from build123d import *

# Parameters (mm, degrees)
SKETCH1_R                                 = 74.5363
SKETCH1_R_2                               = 73.2663
BOSS_EXTRUDE1_DEPTH                       = 19.05
F_1_4_0_25_DIAMETER_HOLE1_REACH           = 179.139
F_1_4_0_25_DIAMETER_HOLE1_BORE_R          = 3.175
F_1_4_0_25_DIAMETER_HOLE1_ON_FACE_2_REACH = 179.139
F_1_4_0_25_DIAMETER_HOLE1_BORE_2_R        = 3.175
F_1_4_0_25_DIAMETER_HOLE4_REACH           = 168.94
F_1_4_0_25_DIAMETER_HOLE4_BORE_R          = 3.175
F_1_4_0_25_DIAMETER_HOLE4_ON_FACE_2_REACH = 168.949
F_1_4_0_25_DIAMETER_HOLE4_BORE_2_R        = 3.175
F_1_4_0_25_DIAMETER_HOLE4_ON_FACE_3_REACH = 168.94
F_1_4_0_25_DIAMETER_HOLE4_BORE_3_R        = 3.175


with BuildPart() as part:
    # Sketch1 → Boss-Extrude1 (new body)
    with BuildSketch(Plane(origin=(0, 0, 0), x_dir=(1, 0, 0), z_dir=(0, 1, 0))):
        with Locations(Location((0, 0, 0), (0, 0, 90))):
            Circle(SKETCH1_R)
        with Locations(Location((0, 0, 0), (0, 0, 90))):
            Circle(SKETCH1_R_2, mode=Mode.SUBTRACT)
    extrude(amount=BOSS_EXTRUDE1_DEPTH)

    # 1/4 (0.25) Diameter Hole1 bore (on position points) → 1/4 (0.25) Diameter Hole1 (cut, up to next)
    with BuildSketch(Plane(origin=(-29.721280226, 9.525, -68.354264822), x_dir=(-0.917060074385, 0, 0.398749068925), z_dir=(-0.398749068925, 0, -0.917060074385)), mode=Mode.PRIVATE) as f_1_4_0_25_diameter_hole1_sk1:
        Circle(F_1_4_0_25_DIAMETER_HOLE1_BORE_R)
    f_1_4_0_25_diameter_hole1_tool1 = extrude(f_1_4_0_25_diameter_hole1_sk1.sketch, amount=-F_1_4_0_25_DIAMETER_HOLE1_REACH, mode=Mode.PRIVATE) & part.part
    add(f_1_4_0_25_diameter_hole1_tool1.solids().sort_by_distance((-29.72128, 9.525, -68.354265))[0], mode=Mode.SUBTRACT)

    # 1/4 (0.25) Diameter Hole1 bore 2 (on position points) → 1/4 (0.25) Diameter Hole1 on face 2 (cut, up to next)
    with BuildSketch(Plane(origin=(29.721280226, 9.525, -68.354264822), x_dir=(-0.917060087762, 0, -0.39874903816), z_dir=(0.39874903816, 0, -0.917060087762)), mode=Mode.PRIVATE) as f_1_4_0_25_diameter_hole1_on_face_2_sk1:
        Circle(F_1_4_0_25_DIAMETER_HOLE1_BORE_2_R)
    f_1_4_0_25_diameter_hole1_on_face_2_tool1 = extrude(f_1_4_0_25_diameter_hole1_on_face_2_sk1.sketch, amount=-F_1_4_0_25_DIAMETER_HOLE1_ON_FACE_2_REACH, mode=Mode.PRIVATE) & part.part
    add(f_1_4_0_25_diameter_hole1_on_face_2_tool1.solids().sort_by_distance((29.72128, 9.525, -68.354265))[0], mode=Mode.SUBTRACT)

    # 1/4 (0.25) Diameter Hole4 bore (on position points) → 1/4 (0.25) Diameter Hole4 (cut, up to next)
    with BuildSketch(Plane(origin=(74.5363, 9.525, 0), x_dir=(0, 0, 1), z_dir=(1, 0, 0)), mode=Mode.PRIVATE) as f_1_4_0_25_diameter_hole4_sk1:
        Circle(F_1_4_0_25_DIAMETER_HOLE4_BORE_R)
    f_1_4_0_25_diameter_hole4_tool1 = extrude(f_1_4_0_25_diameter_hole4_sk1.sketch, amount=-F_1_4_0_25_DIAMETER_HOLE4_REACH, mode=Mode.PRIVATE) & part.part
    add(f_1_4_0_25_diameter_hole4_tool1.solids().sort_by_distance((74.5363, 9.525, 0))[0], mode=Mode.SUBTRACT)

    # 1/4 (0.25) Diameter Hole4 bore 2 (on position points) → 1/4 (0.25) Diameter Hole4 on face 2 (cut, up to next)
    with BuildSketch(Plane(origin=(0, 9.674393406, 74.5363), x_dir=(1, 0, 0), z_dir=(0, 0, 1)), mode=Mode.PRIVATE) as f_1_4_0_25_diameter_hole4_on_face_2_sk1:
        Circle(F_1_4_0_25_DIAMETER_HOLE4_BORE_2_R)
    f_1_4_0_25_diameter_hole4_on_face_2_tool1 = extrude(f_1_4_0_25_diameter_hole4_on_face_2_sk1.sketch, amount=-F_1_4_0_25_DIAMETER_HOLE4_ON_FACE_2_REACH, mode=Mode.PRIVATE) & part.part
    add(f_1_4_0_25_diameter_hole4_on_face_2_tool1.solids().sort_by_distance((0, 9.674393, 74.5363))[0], mode=Mode.SUBTRACT)

    # 1/4 (0.25) Diameter Hole4 bore 3 (on position points) → 1/4 (0.25) Diameter Hole4 on face 3 (cut, up to next)
    with BuildSketch(Plane(origin=(-74.5363, 9.525, 0), x_dir=(0, 0, -1), z_dir=(-1, 0, 0)), mode=Mode.PRIVATE) as f_1_4_0_25_diameter_hole4_on_face_3_sk1:
        Circle(F_1_4_0_25_DIAMETER_HOLE4_BORE_3_R)
    f_1_4_0_25_diameter_hole4_on_face_3_tool1 = extrude(f_1_4_0_25_diameter_hole4_on_face_3_sk1.sketch, amount=-F_1_4_0_25_DIAMETER_HOLE4_ON_FACE_3_REACH, mode=Mode.PRIVATE) & part.part
    add(f_1_4_0_25_diameter_hole4_on_face_3_tool1.solids().sort_by_distance((-74.5363, 9.525, 0))[0], mode=Mode.SUBTRACT)


solid = part.part
Design review of the part built by this model. Coordinates are the model's own, in mm. A direction names the side the tool comes from. Give positions to 0.01 mm unless a question says otherwise; leave off trailing zeros. Loops run counter-clockwise (first coordinate to the right, second up) from the corner with the lowest first, then second, coordinate; pieces in that order, holes last. Notation, with made-up numbers: M -18,36.5 L 13,36.5 A24 ccw 13,65.5 Z; hole C -6,33.25 d6. An arc over 180 degrees is marked long. Answer as a JSON object with one key per item and string values.
Item 1: We need section B-B (z = 0). State the section outline as (x, y) points.
Output values:
{"outline": "M -74.54,0 L -73.27,0 L -73.27,6.35 L -74.54,6.35 Z; M -74.54,12.7 L -73.27,12.7 L -73.27,19.05 L -74.54,19.05 Z; M 73.27,0 L 74.54,0 L 74.54,6.35 L 73.27,6.35 Z; M 73.27,12.7 L 74.54,12.7 L 74.54,19.05 L 73.27,19.05 Z"}
Item 2: For P1, Ø7.5, axis at y = 9.525, z = 0, coming from the -X side; P2, Ø5, axis at x = -56.5, y = 12.5, coming from the +Z side; P3, Ø1.5, axis at y = 13, z = -27, coming from the -X side; P4, Ø6, axis at y = 16, z = 18, coming from the +X side, all flat-tipped, find the tip position at first contact; note any pin that passes through.
Output values:
{"P1": "stops at x = -74.54", "P2": "stops at z = 51.38", "P3": "stops at x = -69.76", "P4": "stops at x = 73.01"}
Item 3: Machinability: for faces 1 (the face through (-49.52, 9.39, 54)), 2 (the face through (2.933, 8.458, 73.876)), which of the approach directions +Z, -Z, +X, -X, +Y, -Y give a long, thin tool a straight path to every point of the face, cutting with its end or side? Answer none if there is none.
Output values:
{"face 1": "+Y, -Y", "face 2": "+Z"}
Item 4: Wall thickness on line 1 along Y through (x, z) = (-73.55, 0); line 2 along Z through (x, y) = (-48, 12); line 3 along Z through (x, y) = (1.5, 2.75): over which ranges is each line inside the solid? List them lowest first.
Output values:
{"line 1": "y = 0 to 6.35, 12.7 to 19.05", "line 2": "z = -57.02 to -55.35, 55.35 to 57.02", "line 3": "z = -74.52 to -73.25, 73.25 to 74.52"}
Item 5: Mouldability with a two-part tool opening along Z and no side actions: class faces 3 (the face through (-32.15, 8.31, -66.58)), 4 (the face through (49, 19.05, -55)), 5 (the face through (-50.375, 9.392, 54.936)) as pulls with the +Z half, pulls with the -Z half, needs draft (parallel to the pull), parting line crosses it, or undercut.
Output values:
{"face 3": "undercut", "face 4": "needs draft", "face 5": "parting line crosses it"}
Item 6: We need section C-C (x = 0). State the section outline as (y, z) points.
Output values:
{"outline": "M 0,-74.54 L 19.05,-74.54 L 19.05,-73.27 L 0,-73.27 Z; M 0,73.27 L 6.5,73.27 L 6.5,74.54 L 0,74.54 Z; M 12.85,73.27 L 19.05,73.27 L 19.05,74.54 L 12.85,74.54 Z"}
Item 7: We need section A-A (x = -56.5). State the section outline as (y, z) points.
Output values:
{"outline": "M 0,-48.61 L 19.05,-48.61 L 19.05,-46.64 L 0,-46.64 Z; M 0,46.64 L 19.05,46.64 L 19.05,48.61 L 0,48.61 Z"}
